Answer from the drawing. Dimensions are ordinates in mm from the lowest x, y and z of the part. Coordinates: 2 decimals unless noted, no trailing zeros. Order: outer loops, then holes, each group sorted by start corner. A loop starts at its lowest first (then second) coordinate and runs counter-clockwise, first axis right, second up. Notation, with made-up numbers: (42.25, -31.5) - (75.25, -31.5) arc R20 ccw to (75.25, -0.5) - close; hole circle Ø10 at (8.5, 31). An arc over 180 degrees is marked (long way). Use CSV: the item, a comma, the result in double quotes. Start each with the question number.
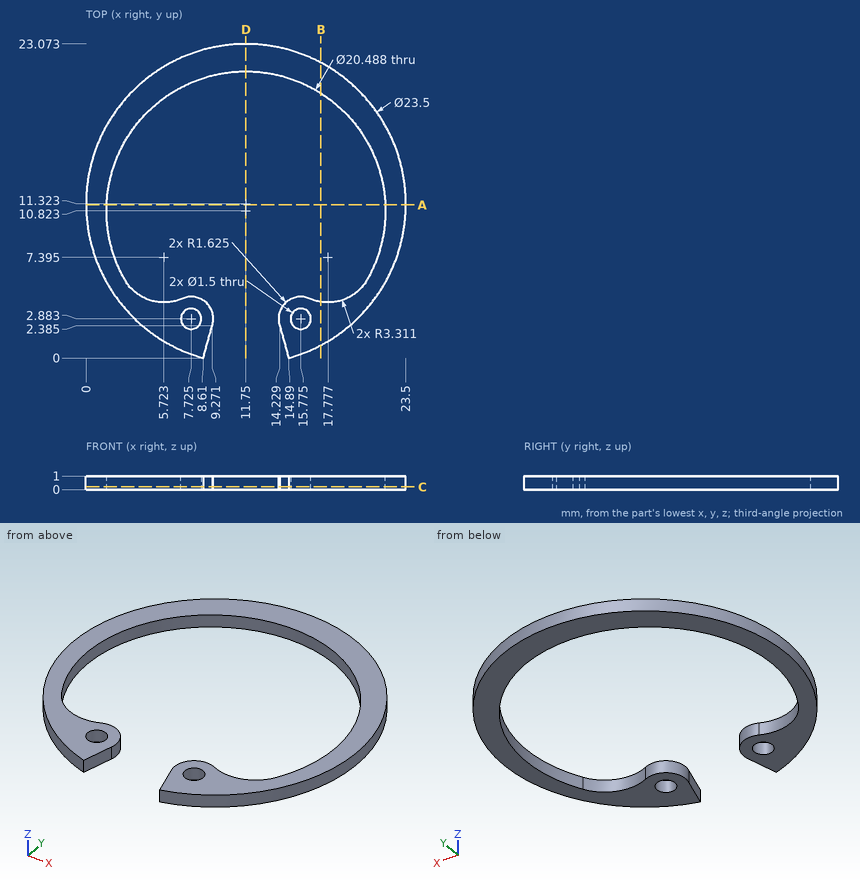
1) The part is cut by section C-C on z = 0.2. State how many separate pieces and enclosed holes the cut face has.
2) Straight lines are drawn through the part: line 1 (X direction, y = 13, z = 0.95); line 2 (X direction, y = 8.5, z = 0.3) (1 decimal); line 3 (Y direction, x = 4.25, z = 0.6) (1 decimal). For each, find the intervals that lie inside material, in ascending order. Write a range as [from, to].
3) The part is cut by section A-A on y = 11.25. Determine the outline of the cut face in (x, z) (1 decimal).
4) The part is cut by section B-B on x = 17.25. Determine the outline of the cut face in (y, z) (1 decimal).
5) The part is cut by section D-D on x = 11.75. Determine the outline of the cut face in (y, z).
Answer key:
1,separate pieces,"1"
1,enclosed holes,"2"
2,line 1,"[0.12, 1.74], [21.76, 23.38]"
2,line 2,"[0.3, 1.8], [21.7, 23.2]"
2,line 3,"[2.3, 4.4], [17.8, 20.4]"
3,outline,"(0, 0) - (1.5, 0) - (1.5, 1) - (0, 1) - close; (22, 0) - (23.5, 0) - (23.5, 1) - (22, 1) - close"
4,outline,"(0.9, 0) - (4.1, 0) - (4.1, 1) - (0.9, 1) - close; (19.5, 0) - (21.7, 0) - (21.7, 1) - (19.5, 1) - close"
5,outline,"(21.07, 0) - (23.07, 0) - (23.07, 1) - (21.07, 1) - close"
